from build123d import *

# Parameters (mm, degrees)
F0_R     = 4.7625
F1_DEPTH = 101.6
F3_DEPTH = 6.35


with BuildPart() as f1:
    # F0 (on Front) → F1 (new body)
    with BuildSketch(Plane.XZ):
        Circle(F0_R)
    extrude(amount=F1_DEPTH)

    # F2 (on Front) → F3 (join)
    with BuildSketch(Plane.XZ):
        Polygon((7.332321, -0.019882), (3.683379, 6.340036), (-3.648942, 6.359918), (-7.332321, 0.019882), (-3.683379, -6.340036), (3.648942, -6.359918), align=None)
    extrude(amount=F3_DEPTH)


solid = f1.part
Geometry: final body of the model. Coordinates: model frame, mm. A direction names the side the tool comes from. Round coordinates to 2 decimals unless told otherwise and drop trailing zeros. Loops run counter-clockwise (first coordinate to the right, second up) from the corner with the lowest first, then second, coordinate; pieces in that order, holes last.
Q1. Material intervals for L1, parallel to Y at x = -2, z = -6; L2, parallel to X at y = -43, z = -0.25; L3, parallel to X at y = -73, z = -3, sorted ascending.
Q2. Access query for faces 1 (the flat face through (5, -6.35, 0)), 2 (the flat face through (-5.465, -3.131, 3.234)). Directions: +Z, -Z, +X, -X, +Y, -Y. A direction counts if a zero-diameter tool reaches every point of the face in a straight line with its end or side. Return the directions, or none.
Q3. Section B-B on z = 2. Return loops of the section in (x, y), plus the area to 3 significant figures.
Q4. Section C-C on y = -13.5. Return loops of the section in (x, z) (1 decimal).
Q5. Section A-A on x = -2.5. Return loops of the section in (y, z).
Q6. Pin query (flat end, axial travel): P1, Ø5, axis at y = -10.5, z = 3, coming from the -X side; P2, Ø6, axis at y = -63, z = 2.5, coming from the +X side; P3, Ø4, axis at y = -57, z = 0, coming from the -X side. Return the tip coordinate at first contact, or that it passes through.
Evaluation:
1. L1: y = -6.35 to 0
1. L2: x = -4.76 to 4.76
1. L3: x = -3.7 to 3.7
2. face 1: -Y
2. face 2: +Z, -X, +Y, -Y
3. outline: (-6.18, -6.35) - (-4.32, -6.35) - (-4.32, -101.6) - (4.32, -101.6) - (4.32, -6.35) - (6.17, -6.35) - (6.17, 0) - (-6.18, 0) - close
3. area: 902 mm2
4. outline: circle Ø9.5 at (0, 0)
5. outline: (-101.6, -4.05) - (-6.35, -4.05) - (-6.35, -6.34) - (0, -6.34) - (0, 6.36) - (-6.35, 6.36) - (-6.35, 4.05) - (-101.6, 4.05) - close
6. P1: stops at x = -4.74
6. P2: stops at x = 4.76
6. P3: stops at x = -4.76
